```python
from build123d import *

# Parameters (mm, degrees)
F3_R     = 2
F4_DEPTH = 25


with BuildPart() as f2:
    # F0 (on Right) → F2 (revolve)
    with BuildSketch(Plane.YZ):
        Polygon((0, 18), (0, 0), (8, 0), (8, 4.5), (3, 4.5), (3, 13), (18, 13), (18, 18), align=None)
    revolve(axis=Axis((0, -0.950184, 0), (0, 1, 0)))

    # F3 (on face) → F4 (cut)
    with BuildSketch(Plane(origin=(0, 8, 0), x_dir=(-1, 0, 0), z_dir=(0, 1, 0))):
        Circle(F3_R)
    extrude(amount=-F4_DEPTH, mode=Mode.SUBTRACT)


solid = f2.part
```
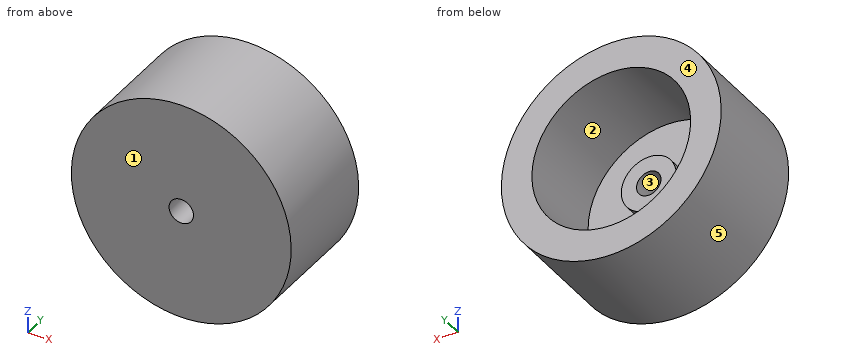
Design review of the part built by this model. Coordinates are the model's own, in mm. Face numbers are marked on the shaded views. A direction names the side the tool comes from. Round coordinates to 2 decimals unless told otherwise and drop trailing zeros. Write each loop counter-clockwise with the first axis right and the second up, starting at its lowest first coordinate (ties: lowest second). Pieces come first, ordered by that corner, then holes. Notation, with made-up numbers: (3.25, -32.5) -> (18.25, -32.5) arc R14 cw to (18.25, -15.5) -> close; hole circle Ø10 at (-15, 60.5). An arc over 180 degrees is marked (long way). Answer in a Markdown table with one row per item.
Q1. Draft analysis for pull direction X (two halves, no side actions). For the marked faces 3, 4 and 5, state which applies: +X half, -X half, draft (parallel to the pull), parting line (faces both ways), or undercut.
The answers:
| item | result |
|---|---|
| face 3 | undercut |
| face 4 | draft |
| face 5 | parting line |
Q2. For the marked faces 1 and 2, list the 3-axis set-ups (+Z, -Z, +X, -X, +Y, -Y) from which the entire face can be reached by the end or side of a thin tool; tool diameter is ignored.
The answers:
| item | result |
|---|---|
| face 1 | +Z, -Z, +X, -X, -Y |
| face 2 | +Y |
Q3. Take a section at B-B, the plane x = 0. State the section outline as (y, z) points, then the cut area to 3 significant figures.
The answers:
| item | result |
|---|---|
| outline | (0, -18) -> (18, -18) -> (18, -13) -> (3, -13) -> (3, -4.5) -> (8, -4.5) -> (8, -2) -> (0, -2) -> close; (0, 2) -> (8, 2) -> (8, 4.5) -> (3, 4.5) -> (3, 13) -> (18, 13) -> (18, 18) -> (0, 18) -> close |
| area | 271 mm² |
Q4. Take a section at C-C, the plane y = 3.5. State the section outline as (x, z) points.
The answers:
| item | result |
|---|---|
| outline | circle Ø36 at (0, 0); circle Ø9 at (0, 0); hole circle Ø26 at (0, 0); hole circle Ø4 at (0, 0) |
Q5. Take a section at D-D, the plane y = 10. State the section outline as (x, z) points.
The answers:
| item | result |
|---|---|
| outline | circle Ø36 at (0, 0); hole circle Ø26 at (0, 0) |
Q6. To check wall thickness, follow L1, parallel to Y at x = 5, z = -0.5; L2, parallel to Z at x = 10, y = 14.25; L3, parallel to Z at x = -8, y = 9.25. State the ranges of each line that lie inside material, in increasing order. Write a range as [from, to].
The answers:
| item | result |
|---|---|
| L1 | [0, 3] |
| L2 | [-14.97, -8.31], [8.31, 14.97] |
| L3 | [-16.12, -10.25], [10.25, 16.12] |
Q7. Take a section at A-A, the plane z = 0. State the section outline as (x, y) points.
The answers:
| item | result |
|---|---|
| outline | (-18, 0) -> (-2, 0) -> (-2, 8) -> (-4.5, 8) -> (-4.5, 3) -> (-13, 3) -> (-13, 18) -> (-18, 18) -> close; (2, 0) -> (18, 0) -> (18, 18) -> (13, 18) -> (13, 3) -> (4.5, 3) -> (4.5, 8) -> (2, 8) -> close |
Q8. Clearance check with flat-ended pins moving along their axes: pin 1 Ø21 at (x, z) = (0, 0) entering from +Y; pin 2 Ø5 at (y, z) = (4.5, 4) entering from -X; pin 3 Ø5 at (y, z) = (7.5, 13.5) entering from -X; pin 4 Ø3.5 at (x, z) = (0, 0) entering from -Y. State where each tip first meets the part, or that it passes through.
The answers:
| item | result |
|---|---|
| pin 1 | y = 8 |
| pin 2 | x = -17.94 |
| pin 3 | x = -14.25 |
| pin 4 | through |
